from build123d import *

# Parameters (mm, degrees)
F0_W        = 175
F0_H        = 88.5
F1_DEPTH    = 85
F2_SIZE     = 17.678
F3_T        = -1
F4_W        = 43
F4_H        = 25
F5_DEPTH    = 2
F6_T1_DEPTH = 1
F7_SIZE     = 4


# Not quite as in the source:
# - a fillet or chamfer that OpenCascade refuses, or shapes differently, is made with other operations: its cross-section is extruded or revolved along the edge and cut away or added


with BuildPart() as f1:
    # F0 (on Top) → F1 (new body)
    with BuildSketch(Plane.XY):
        with Locations((87.5, -44.25)):
            Rectangle(F0_W, F0_H)
    extrude(amount=F1_DEPTH)

    # F2
    f2_edges = [f1.edges().sort_by_distance(p)[0] for p in [
        (87.5, -88.5, 85),
    ]]
    chamfer(f2_edges, length=F2_SIZE)

    # F3
    f3_openings = [f1.faces().sort_by_distance(p)[0] for p in [
        (87.5, -35.411, 85),
    ]]
    offset(amount=F3_T, openings=f3_openings, kind=Kind.INTERSECTION)

    # F4 (on face) → F5 (cut)
    with BuildSketch(Plane.YZ.offset(175)):
        with Locations((-45.25, 52.5)):
            Rectangle(F4_W, F4_H)
    extrude(amount=-F5_DEPTH, mode=Mode.SUBTRACT)

    # F6: chamfer of 4 x 22.6851272785 on 2 edges, made by hand

    # F6_s2 → F6_t1 (join)
    with BuildSketch(Plane.YZ.offset(174)):
        Polygon((-66.75, 61), (-44.0648727215, 65), (-66.75, 65), align=None)
        Polygon((-23.75, 61), (-46.4351272785, 65), (-23.75, 65), align=None)
    extrude(amount=F6_T1_DEPTH)

    # F7
    f7_edges = [f1.edges().sort_by_distance(p)[0] for p in [
        (174.5, -66.75, 40),
        (174.5, -23.75, 40),
    ]]
    chamfer(f7_edges, length=F7_SIZE)


solid = f1.part
Geometry check sheet. Reference: the model listing, model coordinates, mm. A direction names the side the tool comes from. Give positions to 0.01 mm unless a question says otherwise; leave off trailing zeros. Loops run counter-clockwise (first coordinate to the right, second up) from the corner with the lowest first, then second, coordinate; pieces in that order, holes last. Notation, with made-up numbers: (-23, 47.25) -> (36, 47.25) arc R32 ccw to (36, 84.25) -> close; hole circle Ø3 at (43, -20.75). An arc over 180 degrees is marked (long way). Answer in a Markdown table with one row per item. Add a question column.
1) Gauge pin test, flat end, axial feed: P1, Ø5, axis at x = 134.5, z = 70.5, coming from the -Y side. Record the tip position at first contact, or that the pin passes through.
2) Cross-section at B-B on z = 12.5. Record the boundary of the cut face in (x, y), and give its area (3 significant figures).
3) Material ranges on probe 1 along X at (y, z) = (-9.5, 74.5); probe 2 along Y at (x, z) = (151, 49); probe 3 along X at (y, z) = (-27, 59), recorded low to high. Write a range as from..to.
4) Set-up check for faces 4 (the face through (86, -1, 42)), 5 (the face through (86, -87.5, 33)), 6 (the face through (174.51, -64.72, 41.97)): record each of +Z, -Z, +X, -X, +Y, -Y from which the full face is reachable in a straight line by a thin tool's end or side.
5) Draft check along X on faces 1 (the face through (174.49, -56.15, 62.87)), 2 (the face through (0, -45, 42)), 3 (the face through (86.29, -78.33, 76.08)). Enter one of: pulls with the +X half, pulls with the -X half, needs draft (parallel to the pull), parting line crosses it, or undercut.
6) Cross-section at C-C on z = 59. Record the boundary of the cut face in (x, y), and give its area (3 significant figures).
7) Cross-section at A-A on y = -26. Record the boundary of the cut face in (x, z).
8) Cross-section at D-D on x = 102.5. Record the boundary of the cut face in (y, z), and give its area (3 significant figures).
Outcome:
| question | item | result |
|---|---|---|
| 1 | P1 | stops at y = -87.82 |
| 2 | outline | (0, -88.5) -> (175, -88.5) -> (175, 0) -> (0, 0) -> close; hole (1, -87.5) -> (174, -87.5) -> (174, -1) -> (1, -1) -> close |
| 2 | area | 523 mm^2 |
| 3 | probe 1 | x = 0..1, 174..175 |
| 3 | probe 2 | y = -88.5..-87.5, -1..0 |
| 3 | probe 3 | x = 0..1 |
| 4 | face 4 | +Z |
| 4 | face 5 | none |
| 4 | face 6 | +X |
| 5 | face 1 | needs draft |
| 5 | face 2 | pulls with the -X half |
| 5 | face 3 | undercut |
| 6 | outline | (0, -88.5) -> (175, -88.5) -> (175, -66.75) -> (174, -66.75) -> (174, -87.5) -> (1, -87.5) -> (1, -1) -> (174, -1) -> (174, -23.75) -> (175, -23.75) -> (175, 0) -> (0, 0) -> close |
| 6 | area | 480 mm^2 |
| 7 | outline | (0, 0) -> (175, 0) -> (175, 41.75) -> (174, 41.75) -> (174, 1) -> (1, 1) -> (1, 85) -> (0, 85) -> close; (174, 61.4) -> (175, 61.4) -> (175, 85) -> (174, 85) -> close |
| 8 | outline | (-88.5, 0) -> (0, 0) -> (0, 85) -> (-1, 85) -> (-1, 1) -> (-87.5, 1) -> (-87.5, 66.91) -> (-69.41, 85) -> (-70.82, 85) -> (-88.5, 67.32) -> close |
| 8 | area | 264 mm^2 |
